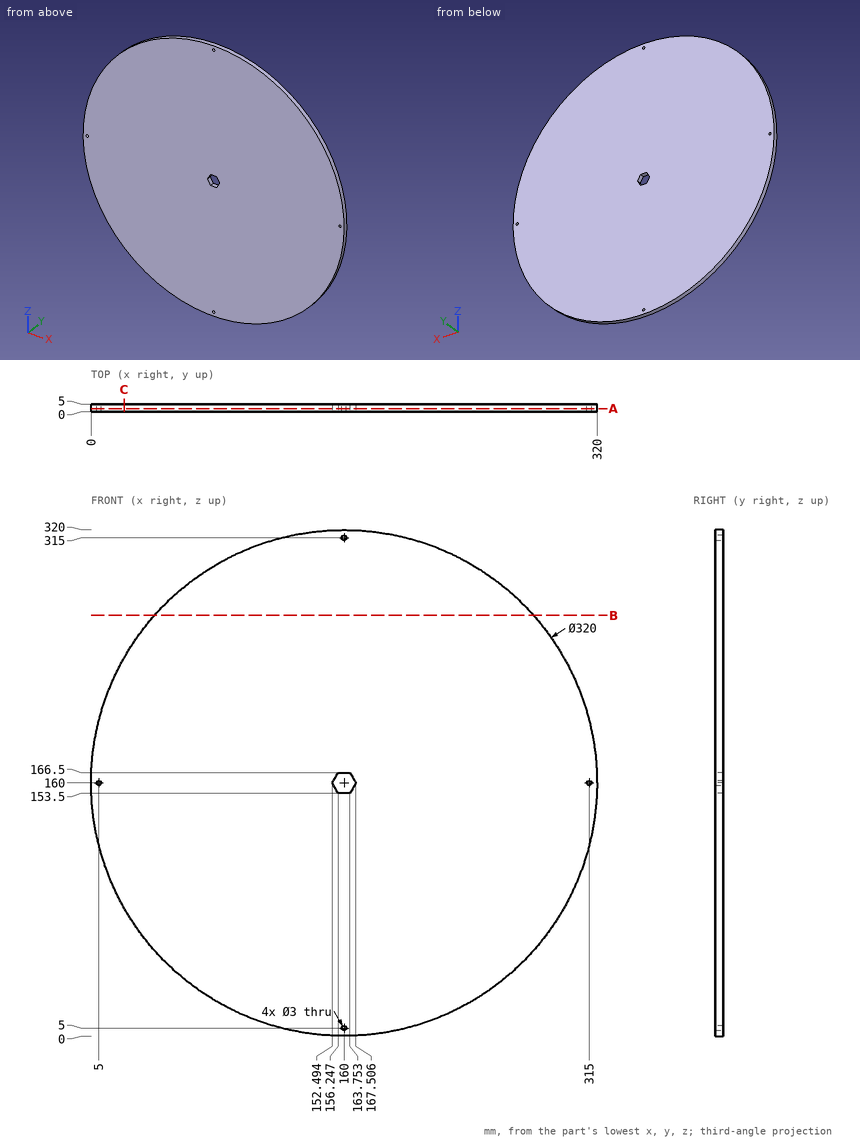
The drawing under review shows one solid part. Ordinate dimensions are in mm from its lowest x, y, z. Coordinates: 2 decimals unless noted, no trailing zeros. Order: outer loops, then holes, each group sorted by start corner. A loop starts at its lowest first (then second) coordinate and runs counter-clockwise, first axis right, second up. Notation, with made-up numbers: (49, 68) -> (63, 68) arc R29 ccw to (63, 92) -> close; hole circle Ø3 at (2.25, 82). An arc over 180 degrees is marked (long way). Answer in a Markdown table with one row per item.
(1) Consider section B-B (z = 266). Write out the cut boundary in (x, y), plus the area to 3 significant figures.
Answers:
| item | result |
|---|---|
| outline | (40.15, 0) -> (279.85, 0) -> (279.85, 5) -> (40.15, 5) -> close |
| area | 1,200 mm² |
(2) Consider section A-A (y = 2). Write out the cut boundary in (x, z) (1 decimal).
Answers:
| item | result |
|---|---|
| outline | circle Ø320 at (160, 160); hole circle Ø3 at (5, 160); hole (152.5, 160) -> (156.2, 153.5) -> (163.8, 153.5) -> (167.5, 160) -> (163.8, 166.5) -> (156.2, 166.5) -> close; hole circle Ø3 at (160, 5); hole circle Ø3 at (160, 315); hole circle Ø3 at (315, 160) |
(3) Consider section C-C (x = 21). Write out the cut boundary in (y, z).
Answers:
| item | result |
|---|---|
| outline | (0, 80.76) -> (5, 80.76) -> (5, 239.24) -> (0, 239.24) -> close |
(4) Insertion check: pin 1 (12 mm diameter, centred on x = 32.5, z = 251, fed in from -Y); pin 2 (3 mm diameter, centred on y = 2.5, z = 213.5, fed in from -X) (1 decimal). Each pin has a flat end and moves straight along its axis. Give the tip position at first contact, or say it passes through.
Answers:
| item | result |
|---|---|
| pin 1 | y = 0 |
| pin 2 | x = 8.7 |
(5) Wall thickness on line 1 along X through (y, z) = (3.3, 160) (1 decimal); line 2 along Z through (x, y) = (172.5, 3.4); line 3 along X through (y, z) = (3.5, 136.5) (1 decimal): over which ranges is each line inside the solid? List them lowest first.
Answers:
| item | result |
|---|---|
| line 1 | 0 to 3.5, 6.5 to 152.5, 167.5 to 313.5, 316.5 to 320 |
| line 2 | 0.49 to 319.51 |
| line 3 | 1.7 to 318.3 |
